Verification items for the finished model (mm, model axes). Give positions to 0.01 mm unless a question says otherwise; leave off trailing zeros. Write each loop counter-clockwise with the first axis right and the second up, starting at its lowest first coordinate (ties: lowest second). Pieces come first, ordered by that corner, then holes. Notation, with made-up numbers: (77.25, -19) -> (102.25, -19) arc R24 cw to (102.25, 20) -> close; hole circle Ø11 at (40.25, -7). An arc over 180 degrees is marked (long way). Use one line per item in the form item = value. Start each with the question number.
(1) Section check A-A, the plane z = 1.25. Record the cut outline in (x, y), plus the area to 3 significant figures.
(2) Depth check by flat-ended pin: pin 1 Ø2 at (y, z) = (75, 5.5) entering from -X. Enter the tip coordinate at first touch or a pass-through.
(3) Scan lines: L1, parallel to Y at x = 5.5, z = 2.75; L2, parallel to Y at x = 6.25, z = 4; L3, parallel to Y at x = 2, z = 5.75 (3 decimals). Record each from-to range of solid material in increasing order.
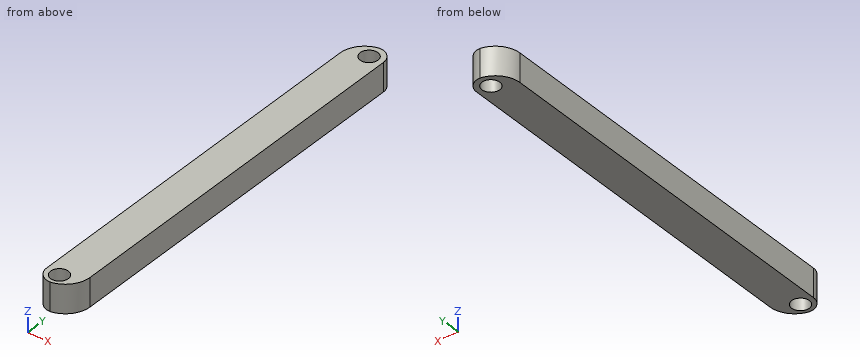
Autodesk Inventor part; units mm, degrees
ref_plane "YZ Plane" through (0, 0, 0) normal (1, 0, 0) x (0, 1, 0)
ref_plane "XZ Plane" through (0, 0, 0) normal (0, 1, 0) x (-1, 0, 0)
ref_plane "XY Plane" through (0, 0, 0) normal (0, 0, 1) x (1, 0, 0)
sketch "Sketch1" plane through (0, 0, 0) normal (0, 0, 1) x (1, 0, 0)
  line L0 (0, 0) -> (10, 0)
  line L1 (10, 0) -> (10, 118.5)
  line L2 (10, 118.5) -> (0, 118.5)
  line L3 (0, 118.5) -> (0, 0)
  dimension "d1" = 10
  dimension "d14" = 118.5
extrude "Extrusion1" add sketch "Sketch1" along normal blind 8
sketch "Sketch2" plane through (0, 0, 8) normal (0, 0, 1) x (1, 0, 0)
  circle A0 centre (3.9473, 3.5528) radius 2.5
  circle A1 centre (6.4473, 196.4185) radius 2.5
  point P0 (0, 0)
  dimension "d4" = 5
  dimension "d5" = 5
extrude "Extrusion2" cut sketch "Sketch2" against normal through all
sketch "Sketch3" plane through (0, 0, 8) normal (0, 0, 1) x (1, 0, 0)
  circle A0 centre (6, 114.5) radius 2.5
  line L0 (10, 118.5) -> (0, 118.5)
  line L1 (10, 0) -> (10, 118.5)
  point P0 (0, 0)
  dimension "d8" = 5
  dimension "d9" = 4
  dimension "d10" = 4
extrude "Extrusion3" cut sketch "Sketch3" against normal through all
fillet "Fillet3" radius 4 2 edges at (10, 118.5, 4) (0, 0, 4)
fillet "Fillet4" radius 7 2 edges at (10, 0, 4) (0, 118.5, 4)
properties part number "rod"
Completed:
q1.outline = (0, 4) arc R4 ccw to (4, 0) arc R7 ccw to (10, 6.93) -> (10, 114.5) arc R4 ccw to (6, 118.5) arc R7 ccw to (0, 111.57) -> close; hole circle Ø5 at (3.95, 3.55); hole circle Ø5 at (6, 114.5)
q1.area = 1,120 mm²
q2.pin_1 = 0
q3.L1 = 0.39 to 1.59, 5.51 to 112.05, 116.95 to 118.41
q3.L2 = 0.73 to 2.58, 4.53 to 112.01, 116.99 to 118.49
q3.L3 = 0.536 to 1.985, 5.121 to 116.471
